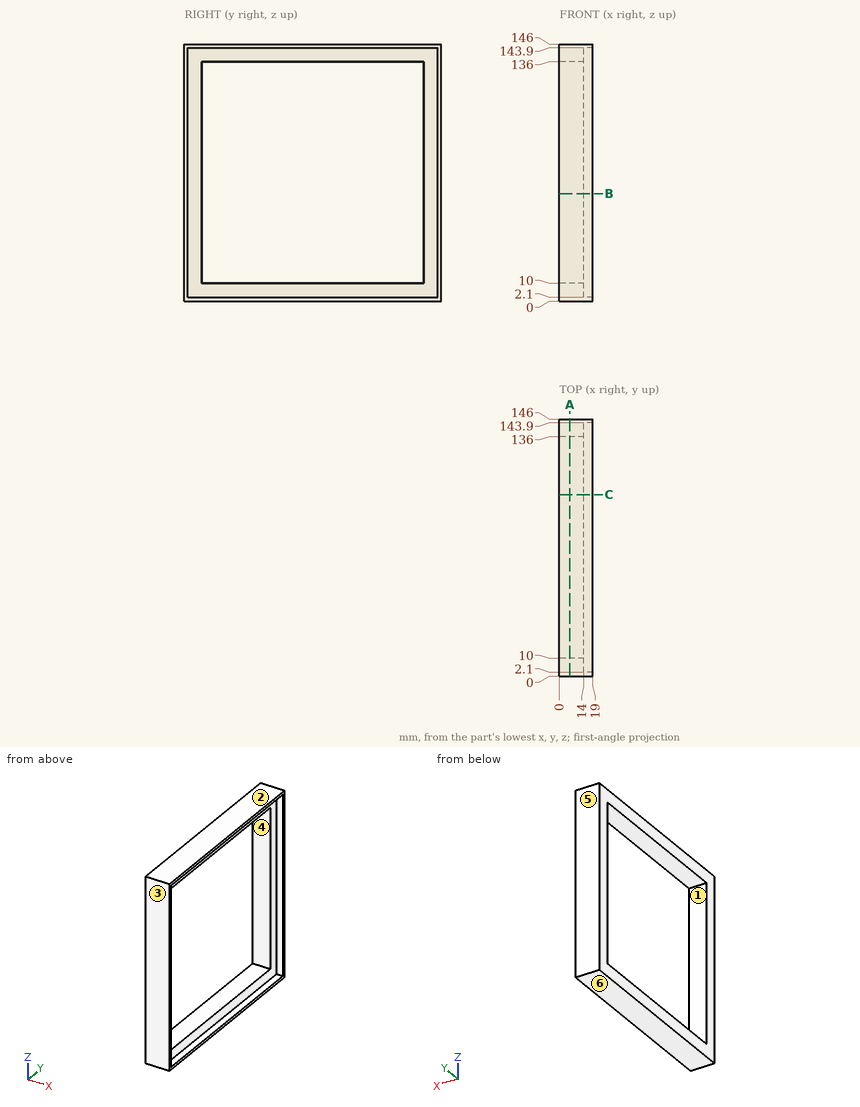
Study the drawing (mm; zero at the part's minimum x, y, z) and answer. A direction names the side the tool comes from. Coordinates: 2 decimals unless noted, no trailing zeros. Loops run counter-clockwise (first coordinate to the right, second up) from the corner with the lowest first, then second, coordinate; pieces in that order, holes last. Notation, with made-up numbers: M 26.25,-25 L 76.25,-25 A18 ccw 76.25,-5 Z; hole C 21,68 d10. An arc over 180 degrees is marked long. Answer in a Markdown table with one row per item. Add a question column.
1. A flat-ended cylindrical pin translates along its axis: P1, Ø4, axis at x = 8, z = 105, coming from the -Y side. Find the tip coordinate at first contact, or state that the pin passes through.
2. The mould has two halves that part along Y. Classify the marked faces 3, 4, 5 and 6: pulls with the +Y half, pulls with the -Y half, needs draft (parallel to the pull), parting line crosses it, or undercut.
3. A tool of negligible diameter and unlimited length cuts with its end or side. For the marked faces 1 and 2, from which of +Z, -Z, +X, -X, +Y, -Y can it reach the whole face along a straight path? Write none if from no direction.
4. Find section A-A, the plane x = 6. Write down the section's boundary in (y, z).
5. Find section B-B, the plane z = 61. Write down the section's boundary in (x, y), then the cut area to 3 significant figures.
6. Consider L1, parallel to Y at x = 6.75, z = 128.5; L2, parallel to Y at x = 17.5, z = 82.5. Determine where each line is inside the solid, lowest interval first.
Reported:
| question | item | result |
|---|---|---|
| 1 | P1 | stops at y = 0 |
| 2 | face 3 | pulls with the -Y half |
| 2 | face 4 | undercut |
| 2 | face 5 | pulls with the +Y half |
| 2 | face 6 | needs draft |
| 3 | face 1 | +X, -X |
| 3 | face 2 | +Z, +X, -X, +Y, -Y |
| 4 | outline | M 0,0 L 146,0 L 146,146 L 0,146 Z; hole M 10,10 L 136,10 L 136,136 L 10,136 Z |
| 5 | outline | M 0,0 L 19,0 L 19,2.1 L 14,2.1 L 14,10 L 0,10 Z; M 0,136 L 14,136 L 14,143.9 L 19,143.9 L 19,146 L 0,146 Z |
| 5 | area | 301 mm^2 |
| 6 | L1 | y = 0 to 10, 136 to 146 |
| 6 | L2 | y = 0 to 2.1, 143.9 to 146 |
